Source: three-view drawing plus pictorial views. Frame: mm from the lowest corner of the part. Give positions to 0.01 mm unless a question says otherwise; leave off trailing zeros. Loops run counter-clockwise (first coordinate to the right, second up) from the corner with the lowest first, then second, coordinate; pieces in that order, holes last. Notation, with made-up numbers: M 59,4.25 L 63,4.25 A38 ccw 63,43.25 Z; hole C 76,-33 d1. An arc over 180 degrees is marked long. Write item = value, one per line.
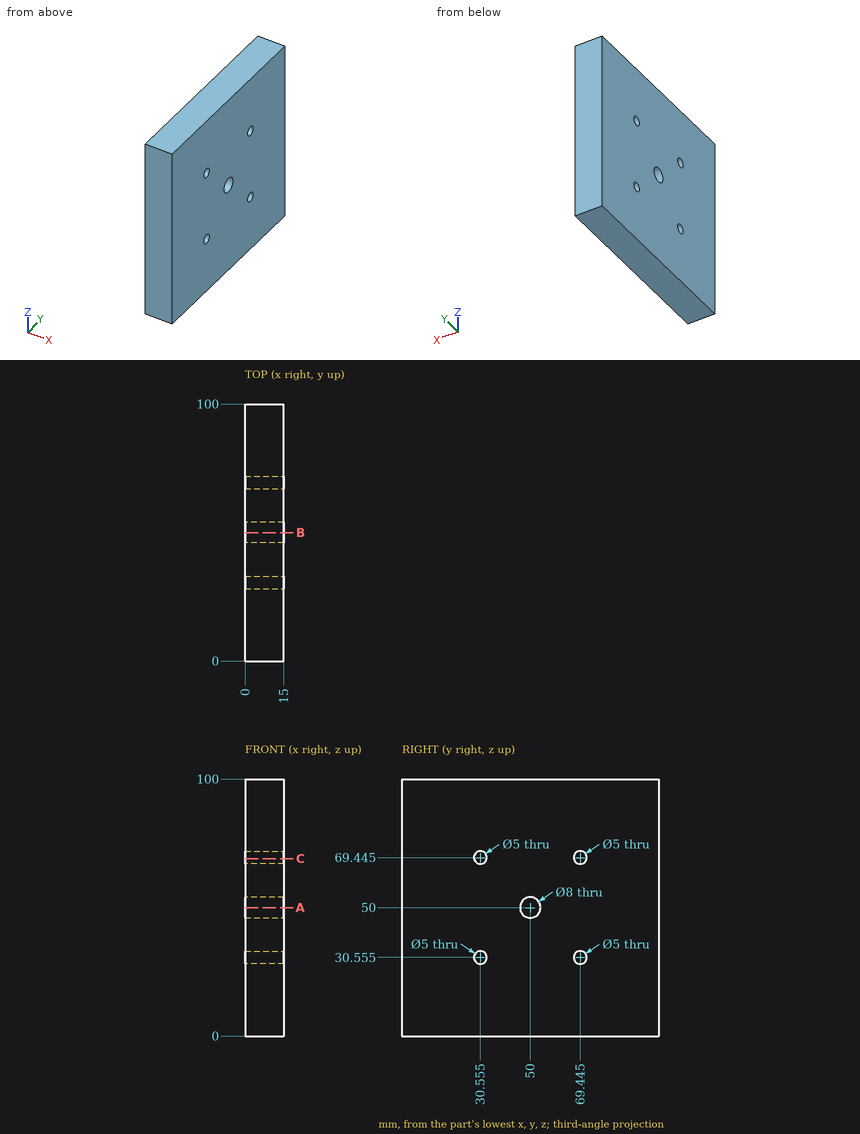
1. Material intervals for probe 1 along Z at (x, y) = (5.25, 30.5) (1 decimal); probe 2 along Z at (x, y) = (13.25, 71) (1 decimal); probe 3 along Y at (x, z) = (12, 50), sorted ascending. Write a range as from..to.
Derived:
probe_1 = 0..28.1, 33.1..66.9, 71.9..100
probe_2 = 0..28.6, 32.5..67.5, 71.4..100
probe_3 = 0..46, 54..100
2. Cut plane A-A, the plane z = 50. Return the cut outline in (x, y), then the cut area to 3 significant figures.
Derived:
outline = M 0,0 L 15,0 L 15,46 L 0,46 Z; M 0,54 L 15,54 L 15,100 L 0,100 Z
area = 1,380 mm²
3. Cut plane C-C, the plane z = 69. Return the cut outline in (x, y) (1 decimal).
Derived:
outline = M 0,0 L 15,0 L 15,28.1 L 0,28.1 Z; M 0,33 L 15,33 L 15,67 L 0,67 Z; M 0,71.9 L 15,71.9 L 15,100 L 0,100 Z
